```python
from build123d import *

# Parameters (mm, degrees)
ESQUISSE1_W              = 8.5
ESQUISSE1_H              = 72
ESQUISSE1_R              = 2.1
BOSS_EXTRU_1_DEPTH       = 17.5
ENL_V_START              = -3
ENL_V_MAT_EXTRU_4_DEPTH  = 3.5
ESQUISSE7_R              = 2.1
BOSS_EXTRU_3_DEPTH       = 8
ESQUISSE3_W              = 8.5
ESQUISSE3_H              = 4
ENL_V_MAT_EXTRU_3_DEPTH  = 19
BOSS_EXTRU_2_START       = -7
BOSS_EXTRU_2_DEPTH       = 12
ESQUISSE8_W              = 8.5
ESQUISSE8_H              = 7
BOSS_EXTRU_4_DEPTH       = 4
ESQUISSE9_R              = 1.6
ENL_V_MAT_EXTRU_5_DEPTH  = 5
ENL_V_START_2            = -4
ESQUISSE10_R             = 1.6
ENL_V_MAT_EXTRU_6_DEPTH  = 2.6
ESQUISSE11_R             = 1.6
ENL_V_MAT_EXTRU_7_DEPTH  = 1.6
ESQUISSE14_W             = 2.5
ESQUISSE14_H             = 10
ENL_V_MAT_EXTRU_9_DEPTH  = 17.6
CHANFREIN1_SIZE          = 0.5
ESQUISSE15_W             = 2.6
ESQUISSE15_H             = 5.7
ESQUISSE15_W_2           = 2.5
ESQUISSE15_H_2           = 10
ESQUISSE15_W_3           = 8.5
ESQUISSE15_H_3           = 15
ENL_V_MAT_EXTRU_10_DEPTH = 10
CHANFREIN2_SIZE          = 9


with BuildPart() as part:
    # Esquisse1 → Boss.-Extru.1 (new body)
    with BuildSketch(Plane.XY):
        with Locations((4.25, 36)):
            Rectangle(ESQUISSE1_W, ESQUISSE1_H)
        with Locations((4, 20.5)):
            Circle(ESQUISSE1_R, mode=Mode.SUBTRACT)
        with Locations((4, 51.5)):
            Circle(ESQUISSE1_R, mode=Mode.SUBTRACT)
    extrude(amount=BOSS_EXTRU_1_DEPTH)

    # Esquisse6 → Enlèv. mat.-Extru.4 (cut)
    with BuildSketch(Plane.XY.offset(17.5).offset(ENL_V_START)):
        Polygon((7.6, 22.578460969), (4, 24.656921938), (0.4, 22.578460969), (0.4, 18.421539031), (4, 16.343078062), (7.6, 18.421539031), align=None)
        Polygon((8.5, 24.656921938), (4, 24.656921938), (7.6, 22.578460969), (7.6, 18.421539031), (4, 16.343078062), (8.5, 16.343078062), align=None)
    enl_v_mat_extru_4 = extrude(amount=-ENL_V_MAT_EXTRU_4_DEPTH, mode=Mode.SUBTRACT)

    # Esquisse7 → Boss.-Extru.3 (add)
    with BuildSketch(Plane(origin=(0, 0, 0), x_dir=(-1, 0, 0), z_dir=(0, 0, -1))):
        with Locations((-4, 20.5)):
            Circle(ESQUISSE7_R)
    boss_extru_3 = extrude(amount=-BOSS_EXTRU_3_DEPTH)

    # Esquisse3 → Enlèv. mat.-Extru.3 (cut)
    with BuildSketch(Plane(origin=(0, 0, 0), x_dir=(-1, 0, 0), z_dir=(0, -1, 0))):
        with Locations((-4.25, -2)):
            Rectangle(ESQUISSE3_W, ESQUISSE3_H)
    enl_v_mat_extru_3 = extrude(amount=-ENL_V_MAT_EXTRU_3_DEPTH, mode=Mode.SUBTRACT)

    # Esquisse5 → Boss.-Extru.2 (add)
    with BuildSketch(Plane.XZ.offset(BOSS_EXTRU_2_START)):
        with BuildLine():
            ThreePointArc((4.662966643, 2.165487935), (4.682946936, 2.27184931), (4.714353535, 2.375413685))
            ThreePointArc((4.714353535, 2.375413685), (5.229781903, 2.78475984), (5.773646598, 2.414028307))
            ThreePointArc((5.773646598, 2.414028307), (5.814751932, 2.291920009), (5.839789089, 2.165534781))
            ThreePointArc((5.839789089, 2.165534781), (5.889607538, 2.072347427), (5.988503907, 2.035128225))
            Line((5.988503907, 2.035128225), (6.514258005, 2.035128225))
            ThreePointArc((6.514258005, 2.035128225), (6.613136609, 2.072331852), (6.662966643, 2.165487935))
            ThreePointArc((6.662966643, 2.165487935), (6.682946936, 2.27184931), (6.714353535, 2.375413685))
            ThreePointArc((6.714353535, 2.375413685), (7.229781903, 2.78475984), (7.773646598, 2.414028307))
            ThreePointArc((7.773646598, 2.414028307), (7.814751932, 2.291920009), (7.839789089, 2.165534781))
            ThreePointArc((7.839789089, 2.165534781), (7.889607538, 2.072347427), (7.988503907, 2.035128225))
            Line((7.988503907, 2.035128225), (8.5, 2.035128225))
            Line((8.5, 2.035128225), (8.5, 4))
            Line((8.5, 4), (0, 4))
            Line((0, 4), (0, 2.035128225))
            Line((0, 2.035128225), (0.514258005, 2.035128225))
            ThreePointArc((0.514258005, 2.035128225), (0.61313661, 2.072331853), (0.662966644, 2.165487937))
            ThreePointArc((0.662966644, 2.165487937), (0.682946936, 2.271849312), (0.714353535, 2.375413685))
            ThreePointArc((0.714353535, 2.375413685), (1.229781903, 2.78475984), (1.773646598, 2.414028307))
            ThreePointArc((1.773646598, 2.414028307), (1.814751932, 2.291920009), (1.839789089, 2.165534781))
            ThreePointArc((1.839789089, 2.165534781), (1.889607538, 2.072347427), (1.988503907, 2.035128225))
            Line((1.988503907, 2.035128225), (2.514258006, 2.035128225))
            ThreePointArc((2.514258006, 2.035128225), (2.613136611, 2.072331854), (2.662966644, 2.16548794))
            ThreePointArc((2.662966644, 2.16548794), (2.682946936, 2.271849313), (2.714353535, 2.375413685))
            ThreePointArc((2.714353535, 2.375413685), (3.229781903, 2.78475984), (3.773646598, 2.414028307))
            ThreePointArc((3.773646598, 2.414028307), (3.814751932, 2.291920009), (3.839789089, 2.165534781))
            ThreePointArc((3.839789089, 2.165534781), (3.889607538, 2.072347427), (3.988503907, 2.035128225))
            Line((3.988503907, 2.035128225), (4.514258005, 2.035128225))
            ThreePointArc((4.514258005, 2.035128225), (4.613136609, 2.072331852), (4.662966643, 2.165487935))
        make_face()
    boss_extru_2 = extrude(amount=-BOSS_EXTRU_2_DEPTH)

    # Esquisse8 → Boss.-Extru.4 (add)
    with BuildSketch(Plane(origin=(0, 0, 4), x_dir=(-1, 0, 0), z_dir=(0, 0, -1))):
        with Locations((-4.25, 3.5)):
            Rectangle(ESQUISSE8_W, ESQUISSE8_H)
    boss_extru_4 = extrude(amount=BOSS_EXTRU_4_DEPTH)

    # Esquisse9 → Enlèv. mat.-Extru.5 (cut)
    with BuildSketch(Plane(origin=(0, 0, 0), x_dir=(-1, 0, 0), z_dir=(0, 0, -1))):
        with Locations((-4.25, 3.75)):
            Circle(ESQUISSE9_R)
        with Locations((-4.25, 22.25)):
            Circle(ESQUISSE9_R)
    enl_v_mat_extru_5 = extrude(amount=-ENL_V_MAT_EXTRU_5_DEPTH, mode=Mode.SUBTRACT)

    # Esquisse10 → Enlèv. mat.-Extru.6 (cut)
    # profile 1 of 4: a face of its own
    with BuildSketch(Plane(origin=(0, 0, 0), x_dir=(-1, 0, 0), z_dir=(0, 0, -1)).offset(ENL_V_START_2)):
        Polygon((-2.604551733, 25.1), (-5.895448267, 25.1), (-7.540896534, 22.25), (-5.895448267, 19.4), (-2.604551733, 19.4), (-0.959103466, 22.25), align=None)
        with Locations((-4.25, 22.25)):
            Circle(ESQUISSE10_R, mode=Mode.SUBTRACT)
    # profile 2 of 4: a face of its own
    with BuildSketch(Plane(origin=(0, 0, 0), x_dir=(-1, 0, 0), z_dir=(0, 0, -1)).offset(ENL_V_START_2)):
        Polygon((-2.604551733, 6.6), (-5.895448267, 6.6), (-7.540896534, 3.75), (-5.895448267, 0.9), (-2.604551733, 0.9), (-0.959103466, 3.75), align=None)
    # profile 3 of 4: a face of its own
    with BuildSketch(Plane(origin=(0, 0, 0), x_dir=(-1, 0, 0), z_dir=(0, 0, -1)).offset(ENL_V_START_2)):
        Polygon((-8.5, 6.6), (-5.895448267, 6.6), (-7.540896534, 3.75), (-5.895448267, 0.9), (-8.5, 0.9), align=None)
    # profile 4 of 4: a face of its own
    with BuildSketch(Plane(origin=(0, 0, 0), x_dir=(-1, 0, 0), z_dir=(0, 0, -1)).offset(ENL_V_START_2)):
        Polygon((-7.540896534, 22.25), (-5.895448267, 25.1), (-8.5, 25.1), (-8.5, 19.4), (-5.895448267, 19.4), align=None)
    enl_v_mat_extru_6 = extrude(amount=-ENL_V_MAT_EXTRU_6_DEPTH, mode=Mode.SUBTRACT)

    # Esquisse11 → Enlèv. mat.-Extru.7 (cut)
    with BuildSketch(Plane(origin=(0, 0, 5), x_dir=(-1, 0, 0), z_dir=(0, 0, -1))):
        with Locations((-4.25, 22.25)):
            Circle(ESQUISSE11_R)
    enl_v_mat_extru_7 = extrude(amount=-ENL_V_MAT_EXTRU_7_DEPTH, mode=Mode.SUBTRACT)

    # Esquisse14 → Enlèv. mat.-Extru.9 (cut)
    with BuildSketch(Plane(origin=(8.5, 0, 0), x_dir=(0, 0, -1), z_dir=(1, 0, 0))):
        with Locations((-6.75, 13)):
            Rectangle(ESQUISSE14_W, ESQUISSE14_H)
    enl_v_mat_extru_9 = extrude(amount=-ENL_V_MAT_EXTRU_9_DEPTH, mode=Mode.SUBTRACT)

    # Symétrie14: Enlèv. mat.-Extru.4, Boss.-Extru.3, Enlèv. mat.-Extru.3, Boss.-Extru.2, Boss.-Extru.4, Enlèv. mat.-Extru.5, Enlèv. mat.-Extru.6, Enlèv. mat.-Extru.7, Enlèv. mat.-Extru.9 across plane
    add(enl_v_mat_extru_4.mirror(Plane(origin=(0, 36, 0), x_dir=(0, 0, 1), z_dir=(0, -1, 0))), mode=Mode.SUBTRACT)
    add(boss_extru_3.mirror(Plane(origin=(0, 36, 0), x_dir=(0, 0, 1), z_dir=(0, -1, 0))))
    add(enl_v_mat_extru_3.mirror(Plane(origin=(0, 36, 0), x_dir=(0, 0, 1), z_dir=(0, -1, 0))), mode=Mode.SUBTRACT)
    add(boss_extru_2.mirror(Plane(origin=(0, 36, 0), x_dir=(0, 0, 1), z_dir=(0, -1, 0))))
    add(boss_extru_4.mirror(Plane(origin=(0, 36, 0), x_dir=(0, 0, 1), z_dir=(0, -1, 0))))
    add(enl_v_mat_extru_5.mirror(Plane(origin=(0, 36, 0), x_dir=(0, 0, 1), z_dir=(0, -1, 0))), mode=Mode.SUBTRACT)
    add(enl_v_mat_extru_6.mirror(Plane(origin=(0, 36, 0), x_dir=(0, 0, 1), z_dir=(0, -1, 0))), mode=Mode.SUBTRACT)
    add(enl_v_mat_extru_7.mirror(Plane(origin=(0, 36, 0), x_dir=(0, 0, 1), z_dir=(0, -1, 0))), mode=Mode.SUBTRACT)
    add(enl_v_mat_extru_9.mirror(Plane(origin=(0, 36, 0), x_dir=(0, 0, 1), z_dir=(0, -1, 0))), mode=Mode.SUBTRACT)

    # Chanfrein1
    chanfrein1_edges = [part.edges().sort_by_distance(p)[0] for p in [
        (1.9, 51.5, 14.5),
        (1.9, 51.5, 11),
        (1.9, 20.5, 11),
        (1.9, 20.5, 14.5),
    ]]
    chamfer(chanfrein1_edges, length=CHANFREIN1_SIZE)

    # Esquisse15 → Enlèv. mat.-Extru.10 (cut)
    # profile 1 of 2: a face of its own
    with BuildSketch(Plane(origin=(8.5, 0, 0), x_dir=(0, 0, -1), z_dir=(1, 0, 0))):
        Polygon((-9, 26), (0, 26), (0, 53), (-2.035128225, 53), (-2.035128225, 65), (0, 65), (0, 72), (-9, 72), (-9, 57), align=None)
        with Locations((-5.3, 49.75)):
            Rectangle(ESQUISSE15_W, ESQUISSE15_H, mode=Mode.SUBTRACT)
        with Locations((-6.75, 59)):
            Rectangle(ESQUISSE15_W_2, ESQUISSE15_H_2, mode=Mode.SUBTRACT)
        with Locations((-5.3, 68.25)):
            Rectangle(ESQUISSE15_W, ESQUISSE15_H, mode=Mode.SUBTRACT)
    # profile 2 of 2: a face of its own
    with BuildSketch(Plane(origin=(8.5, 0, 0), x_dir=(0, 0, -1), z_dir=(1, 0, 0))):
        with Locations((-13.25, 64.5)):
            Rectangle(ESQUISSE15_W_3, ESQUISSE15_H_3)
    extrude(amount=-ENL_V_MAT_EXTRU_10_DEPTH, mode=Mode.SUBTRACT)


with BuildPart() as enl_v_mat_extru_10_kept_piece:
    # of the separate pieces the step leaves, the one the design keeps (enl_v_mat_extru_10_pieces_kept)
    add(part.part.solids().sort_by_distance((6.6, 20.5, 14.5))[0])

    # Chanfrein2
    chanfrein2_edges = [enl_v_mat_extru_10_kept_piece.edges().sort_by_distance(p)[0] for p in [
        (4.25, 26, 9),
    ]]
    chamfer(chanfrein2_edges, length=CHANFREIN2_SIZE - 0.0001)  # a hair under: the kernel refuses the full size


solid = enl_v_mat_extru_10_kept_piece.part
```
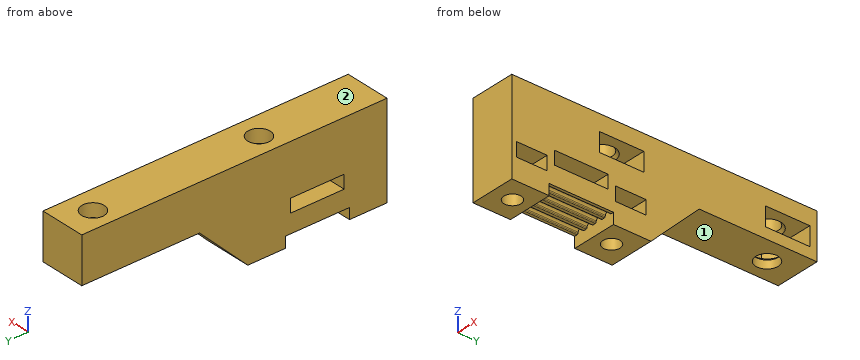
Check sheet for the modelled part. Datum: model origin and axes. Units: mm. Face numbers are marked on the shaded views. A direction names the side the tool comes from. Round coordinates to 2 decimals unless told otherwise and drop trailing zeros. Order: outer loops, then holes, each group sorted by start corner. A loop starts at its lowest first (then second) coordinate and runs counter-clockwise, first axis right, second up.
1) Go/stop test with flat-tipped pins: pin 1 Ø2.5 at (x, y) = (2, 14.5) entering from -Z; pin 2 Ø1.3 at (x, z) = (5.5, 6) entering from +Y; pin 3 Ø5 at (x, y) = (3, 35.5) entering from -Z. Record where each tip stops, or that it passes through.
2) Section check C-C (z = 5). Record the boundary of the cut face in (x, y).
3) Section check D-D (y = 27). Record the boundary of the cut face in (x, z).
4) Section check B-B (z = 16.25). Record the boundary of the cut face in (x, y).
5) Section check A-A (y = 51.5). Record the boundary of the cut face in (x, z).
6) Tool access check on the marked faces 1 and 2. Record the directions out of +Z, -Z, +X, -X, +Y, -Y that give a thin tool (end or side, any length) a straight path to the whole face; none if there is none.
7) Scan lines: line 1 (Z direction, x = 4.25, y = 17.5); line 2 (Y direction, x = 4, z = 9.5); line 3 (Y direction, x = 6, z = 13.25). Record each from-to range of solid material in increasing order.
Result:
1. pin 1: stops at z = 2.04
1. pin 2: stops at y = 32.65
1. pin 3: stops at z = 7
2. outline: (0, 0) - (8.5, 0) - (8.5, 0.9) - (2.6, 0.9) - (0.96, 3.75) - (2.6, 6.6) - (8.5, 6.6) - (8.5, 19.4) - (2.6, 19.4) - (0.96, 22.25) - (2.6, 25.1) - (8.5, 25.1) - (8.5, 31) - (0, 31) - close
3. outline: (0, 1) - (8.5, 1) - (8.5, 17.5) - (0, 17.5) - close
4. outline: (0, 0) - (8.5, 0) - (8.5, 57) - (0, 57) - close; hole circle Ø4.2 at (4, 20.5); hole circle Ø4.2 at (4, 51.5)
5. outline: (0, 9) - (1.9, 9) - (1.9, 10.5) - (1.4, 11) - (0.4, 11) - (0.4, 14.5) - (1.4, 14.5) - (1.9, 15) - (1.9, 17.5) - (0, 17.5) - close; (6.1, 9) - (8.5, 9) - (8.5, 11) - (6.6, 11) - (6.1, 10.5) - close; (6.1, 15) - (6.6, 14.5) - (8.5, 14.5) - (8.5, 17.5) - (6.1, 17.5) - close
6. face 1: -Z, +X, -X, +Y
6. face 2: +Z, +X, -X, +Y, -Y
7. line 1: z = 2.04 to 5.5, 8 to 11, 14.5 to 17.5
7. line 2: y = 0 to 18.4, 22.6 to 49.4, 53.6 to 57
7. line 3: y = 0 to 16.34, 24.66 to 47.34, 55.66 to 57
